Build history of the part. All positions in model axes, mm. Round coordinates to 2 decimals unless told otherwise and drop trailing zeros. Write each loop counter-clockwise with the first axis right and the second up, starting at its lowest first coordinate (ties: lowest second). Pieces come first, ordered by that corner, then holes. Notation, with made-up numbers: (-9, 67) - (36, 67) arc R21 cw to (36, 91) - close; hole circle Ø5 at (47.25, 41.5). An arc over 180 degrees is marked (long way). Write each question's results on one line, items separated by ' | '.
from build123d import *

# Parameters (mm, degrees)
BOSS_EXTRUDE1_DEPTH = 6
FILLET1_R           = 3
SKETCH2_R           = 1.5
CUT_EXTRUDE1_DEPTH  = 121.565334985


with BuildPart() as part:
    # Sketch1 → Boss-Extrude1 (new body)
    with BuildSketch(Plane(origin=(0, 0, 0), x_dir=(1, 0, 0), z_dir=(0, 1, 0))):
        Polygon((0, 0), (51.961524227, 90), (0, 90), (-80, 90), (-80, 0), align=None)
    extrude(amount=BOSS_EXTRUDE1_DEPTH)

    # Fillet1
    fillet1_edges = [part.edges().sort_by_distance(p)[0] for p in [
        (25.980762114, 0, -45),
    ]]
    fillet(fillet1_edges, radius=FILLET1_R)

    # Sketch2 → Cut-Extrude1 (cut, through all)
    with BuildSketch(Plane(origin=(0, 6, 0), x_dir=(1, 0, 0), z_dir=(0, 1, 0))):
        with Locations(Location((-50, 77.5, 0), (0, 0, 270))):
            Circle(SKETCH2_R)
        with Locations(Location((-20, 77.5, 0), (0, 0, 270))):
            Circle(SKETCH2_R)
    extrude(amount=-CUT_EXTRUDE1_DEPTH, mode=Mode.SUBTRACT)


solid = part.part
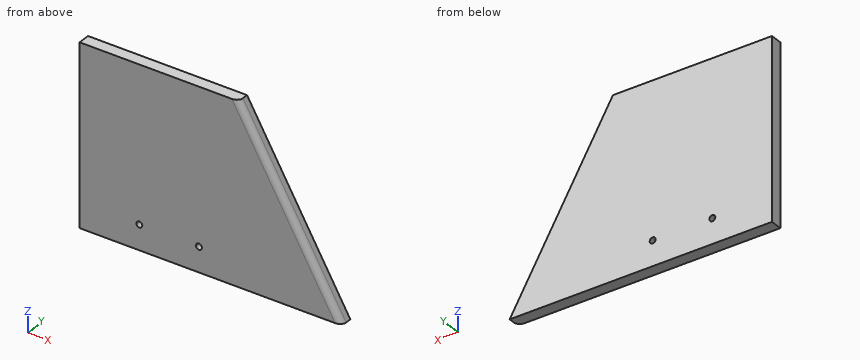
(1) Slice it at A-A, the plane x = -50. Write the cut outline in (y, z).
Worked answers:
outline: (0, -90) - (6, -90) - (6, -79) - (0, -79) - close; (0, -76) - (6, -76) - (6, 0) - (0, 0) - close
(2) Drill centre lines: probe 1 along X at (y, z) = (2.75, -77.5); probe 2 along Z at (x, y) = (-51, 0.4); probe 3 along Z at (x, y) = (19, 1.35). Where is each one in solid material? Low to high. Write a range as [from, to].
Worked answers:
probe 1: x = [-80, -51.5], [-48.5, -21.5], [-18.5, 44.73] | probe 2: z = [-90, -78.62], [-76.38, 0] | probe 3: z = [-90, -33.9]
(3) Slice it at B-B, the plane y = 2. Write the cut outline in (x, z), and give its area (3 significant figures).
Worked answers:
outline: (-80, -90) - (51.76, -90) - (-0.2, 0) - (-80, 0) - close; hole circle Ø3 at (-50, -77.5); hole circle Ø3 at (-20, -77.5) | area: 9,510 mm2
(4) Slice it at C-C, the plane z = -77.5. State how many separate pieces and enclosed holes the cut face has, and give its area (3 significant figures).
Worked answers:
separate pieces: 3 | enclosed holes: 0 | area: 710 mm2
(5) Flat gauge pins, fed straight in: pin 1 Ø2 at (y, z) = (5, -58.5) entering from +X; pin 2 Ø2.5 at (x, z) = (-20, -77.5) entering from +Y; pin 3 Ø2 at (y, z) = (5, -38) entering from +X. Where does each tip first touch, or does it go through?
Worked answers:
pin 1: stops at x = 34.35 | pin 2: passes through | pin 3: stops at x = 22.52
